```python
from build123d import *

# Parameters (mm, degrees)
SKETCH1_W           = 177.8
SKETCH1_H           = 48.26
SKETCH1_W_2         = 4.572
SKETCH1_H_2         = 12.7
BOSS_EXTRUDE1_DEPTH = 4.572
CUT_EXTRUDE1_DEPTH  = 5.08


with BuildPart() as part:
    # Sketch1 → Boss-Extrude1 (new body)
    with BuildSketch(Plane(origin=(0, 0, 0), x_dir=(1, 0, 0), z_dir=(0, 1, 0))):
        with Locations((88.9, 24.13)):
            Rectangle(SKETCH1_W, SKETCH1_H)
        with Locations((162.814, 24.13)):
            Rectangle(SKETCH1_W_2, SKETCH1_H_2, mode=Mode.SUBTRACT)
        with Locations((89.408, 24.13)):
            Rectangle(SKETCH1_W_2, SKETCH1_H_2, mode=Mode.SUBTRACT)
        with Locations((21.336, 24.13)):
            Rectangle(SKETCH1_W_2, SKETCH1_H_2, mode=Mode.SUBTRACT)
    extrude(amount=BOSS_EXTRUDE1_DEPTH)

    # Sketch2 → Cut-Extrude1 (cut)
    with BuildSketch(Plane(origin=(0, 4.572, 0), x_dir=(1, 0, 0), z_dir=(0, 1, 0))):
        with BuildLine():
            Line((49.022, 27.305), (61.722, 27.305))
            ThreePointArc((61.722, 27.305), (64.897, 24.13), (61.722, 20.955))
            Line((61.722, 20.955), (49.022, 20.955))
            ThreePointArc((49.022, 20.955), (45.847, 24.13), (49.022, 27.305))
        make_face()
        with BuildLine():
            Line((117.094, 27.305), (129.794, 27.305))
            ThreePointArc((129.794, 27.305), (132.969, 24.13), (129.794, 20.955))
            Line((129.794, 20.955), (117.094, 20.955))
            ThreePointArc((117.094, 20.955), (113.919, 24.13), (117.094, 27.305))
        make_face()
    extrude(amount=-CUT_EXTRUDE1_DEPTH, mode=Mode.SUBTRACT)


solid = part.part
```
Can you work these out from the model? Positions are in its coordinate system, mm. A direction names the side the tool comes from. Give positions to 0.01 mm unless a question says otherwise; leave off trailing zeros. Order: outer loops, then holes, each group sorted by start corner. A loop starts at its lowest first (then second) coordinate and runs counter-clockwise, first axis right, second up. Notation, with made-up numbers: (79, 81) - (116, 81) arc R34 ccw to (116, 114) - close; hole circle Ø11 at (83.25, 8.5). An arc over 180 degrees is marked (long way). Use a Markdown table: item, result. Add a question column.
Q1. Please list where these lines run through material, in increasing order: line 1 along Z through (x, y) = (58, 4) (3 decimals); line 2 along Z through (x, y) = (165, 0.35); line 3 along X through (y, z) = (3, -27).
Q2. If we section it at C-C on y = 1.35: Write out the boundary of the cut face in (x, z) (3 decimals).
Q3. On a 3-axis mill with a long thin cutter (end or side, diameter ignored), from which of +Z, -Z, +X, -X, +Y, -Y can I reach the whole of each face in a straight line? I mean faces 5 (the flat face through (88, 2, 0)), 6 (the cylindrical face through (113.92, 2.32, -24.06)). Say none if no direction works.
Q4. If we mould it in two halves opening along Z, with no side actions, what happens to faces 1 (the flat face through (21, 2, -17.78)), 2 (the cylindrical face through (45.848, 2.318, -24.06)), 3 (the flat face through (88, 4.572, -35)), 4 (the flat face through (88, 2, -48.26))? For each: released by +Z, released by -Z, zero draft, split by the parting line, or undercut.
Q5. If we section it at B-B on z = -24.13: Write out the boundary of the cut face in (x, y), plus the area to 3 significant figures.
Q6. If we section it at A-A on x = 50.5: Write out the boundary of the cut face in (y, z) (3 decimals), plus the area to 3 significant figures.
Q7. I'm going to push a flat-ended pin straight in: pin 1 (1.5 mm diameter, centred on x = 156, y = 1.5, fed in from +Z). Where does the tip first touch, or does it pass through?
Answers follow:
| question | item | result |
|---|---|---|
| 1 | line 1 | z = -48.26 to -27.305, -20.955 to 0 |
| 1 | line 2 | z = -48.26 to -30.48, -17.78 to 0 |
| 1 | line 3 | x = 0 to 19.05, 23.62 to 47.66, 63.08 to 87.12, 91.69 to 115.74, 131.15 to 160.53, 165.1 to 177.8 |
| 2 | outline | (0, -48.26) - (177.8, -48.26) - (177.8, 0) - (0, 0) - close; hole (19.05, -30.48) - (23.622, -30.48) - (23.622, -17.78) - (19.05, -17.78) - close; hole (49.022, -27.305) - (61.722, -27.305) arc R3.175 ccw to (61.722, -20.955) - (49.022, -20.955) arc R3.175 ccw to start; hole (87.122, -30.48) - (91.694, -30.48) - (91.694, -17.78) - (87.122, -17.78) - close; hole (117.094, -27.305) - (129.794, -27.305) arc R3.175 ccw to (129.794, -20.955) - (117.094, -20.955) arc R3.175 ccw to start; hole (160.528, -30.48) - (165.1, -30.48) - (165.1, -17.78) - (160.528, -17.78) - close |
| 3 | face 5 | +Z, +X, -X, +Y, -Y |
| 3 | face 6 | +Y, -Y |
| 4 | face 1 | undercut |
| 4 | face 2 | undercut |
| 4 | face 3 | zero draft |
| 4 | face 4 | released by -Z |
| 5 | outline | (0, 0) - (19.05, 0) - (19.05, 4.57) - (0, 4.57) - close; (23.62, 0) - (45.85, 0) - (45.85, 4.57) - (23.62, 4.57) - close; (64.9, 0) - (87.12, 0) - (87.12, 4.57) - (64.9, 4.57) - close; (91.69, 0) - (113.92, 0) - (113.92, 4.57) - (91.69, 4.57) - close; (132.97, 0) - (160.53, 0) - (160.53, 4.57) - (132.97, 4.57) - close; (165.1, 0) - (177.8, 0) - (177.8, 4.57) - (165.1, 4.57) - close |
| 5 | area | 576 mm^2 |
| 6 | outline | (0, -48.26) - (4.572, -48.26) - (4.572, -27.305) - (0, -27.305) - close; (0, -20.955) - (4.572, -20.955) - (4.572, 0) - (0, 0) - close |
| 6 | area | 192 mm^2 |
| 7 | pin 1 | stops at z = 0 |
